Here's how the part is built. I have some questions about the finished solid (model axes, mm). A direction names the side the tool comes from. Give positions to 0.01 mm unless a question says otherwise; leave off trailing zeros. Write each loop counter-clockwise with the first axis right and the second up, starting at its lowest first coordinate (ties: lowest second). Pieces come first, ordered by that corner, then holes. Notation, with made-up numbers: (41, -40) -> (67, -40) arc R17 ccw to (67, -29) -> close; hole circle Ø8 at (70, 25). An arc over 180 degrees is marked (long way). Use CSV: the item, a comma, the result in double quotes. Start each with the question number.
(1) Suppose I cut it at C-C on x = 6.5. List the corners of the cut face in (y, z) for me, plus the area to 3 significant figures.
(2) Suppose I cut it at D-D on z = 2. Give the number of separate pieces and of enclosed holes in the cut face, plus the area to 3 significant figures.
(3) If we mould it in two halves opening along X, with no side actions, what happens to faces 3 (the flat face through (-21.8, -31, 13)), 4 (the flat face through (0, -77.62, 13)), 5 (the flat face through (9, 7.62, 13))? For each: pulls with the +X half, pulls with the -X half, needs draft (parallel to the pull), parting line crosses it, or undercut.
(4) Suppose I cut it at A-A on y = -5.5. List the corners of the cut face in (x, z) for me.
(5) Suppose I cut it at B-B on y = -34. List the corners of the cut face in (x, z) for me, plus the area to 3 significant figures.
(6) Which directions (+Z, -Z, +X, -X, +Y, -Y) give clear straight access to the entire face, cutting with the end or side of a thin tool? Please do faces 1 (the flat face through (9.73, -37.21, 12.52)), 2 (the flat face through (0, 13.97, 13)).
(7) I need wall thicknesses on L1, parallel to X at y = -56.5, z = 21; L2, parallel to Y at x = -13, z = 4; L3, parallel to X at y = 4, z = 7. Which ranges of each line are inside material? Lowest first, please. Write a range as [from, to].
from build123d import *

# Parameters (mm, degrees)
BOSS_EXTRUDE1_DEPTH = 25.4
FILLET1_R           = 0.762


with BuildPart() as part:
    # Sketch1 → Boss-Extrude1 (new body)
    with BuildSketch(Plane.XY):
        Polygon((-21.799999961, -13.97), (-21.799999961, 13.97), (21.799999961, 13.97), (21.799999961, -13.97), (21.799999961, -77.619999954), (-21.799999961, -77.619999954), align=None)
        Polygon((-15.449999961, 7.62), (-2.54, 7.62), (-2.54, 4.572), (-6.6548, 4.572), (-2.933726616, 0.762), (2.933726616, 0.762), (6.6548, 4.572), (2.54, 4.572), (2.54, 7.62), (15.449999961, 7.62), (15.449999961, -7.62), (-15.449999961, -7.62), align=None, mode=Mode.SUBTRACT)
        Polygon((-13.601813914, -20.32), (0, -40.176776526), (13.601813914, -20.32), align=None, mode=Mode.SUBTRACT)
        Polygon((15.449999961, -28.858349607), (3.848460993, -45.794999977), (15.449999961, -62.731650347), align=None, mode=Mode.SUBTRACT)
        Polygon((-3.848460993, -45.794999977), (-15.449999961, -62.731650347), (-15.449999961, -28.858349607), align=None, mode=Mode.SUBTRACT)
        Polygon((0, -51.413223428), (-13.601813914, -71.269999954), (13.601813914, -71.269999954), align=None, mode=Mode.SUBTRACT)
    extrude(amount=BOSS_EXTRUDE1_DEPTH)

    # Fillet1
    fillet1_edges = [part.edges().sort_by_distance(p)[0] for p in [
        (2.54, 7.62, 12.7),
        (2.54, 4.572, 12.7),
        (6.6548, 4.572, 12.7),
        (2.933726616, 0.762, 12.7),
        (-2.933726616, 0.762, 12.7),
        (-6.6548, 4.572, 12.7),
        (-2.54, 4.572, 12.7),
        (-2.54, 7.62, 12.7),
    ]]
    fillet(fillet1_edges, radius=FILLET1_R)


solid = part.part
Geometry says:
1,outline,"(-77.62, 0) -> (-71.27, 0) -> (-71.27, 25.4) -> (-77.62, 25.4) -> close; (-60.9, 0) -> (-49.67, 0) -> (-49.67, 25.4) -> (-60.9, 25.4) -> close; (-41.92, 0) -> (-30.69, 0) -> (-30.69, 25.4) -> (-41.92, 25.4) -> close; (-20.32, 0) -> (-7.62, 0) -> (-7.62, 25.4) -> (-20.32, 25.4) -> close; (7.62, 0) -> (13.97, 0) -> (13.97, 25.4) -> (7.62, 25.4) -> close"
1,area,"1,220 mm²"
2,separate pieces,"1"
2,enclosed holes,"5"
2,area,"2,640 mm²"
3,face 3,"pulls with the -X half"
3,face 4,"needs draft"
3,face 5,"undercut"
4,outline,"(-21.8, 0) -> (-15.45, 0) -> (-15.45, 25.4) -> (-21.8, 25.4) -> close; (15.45, 0) -> (21.8, 0) -> (21.8, 25.4) -> (15.45, 25.4) -> close"
5,outline,"(-21.8, 0) -> (-15.45, 0) -> (-15.45, 25.4) -> (-21.8, 25.4) -> close; (-11.93, 0) -> (-4.23, 0) -> (-4.23, 25.4) -> (-11.93, 25.4) -> close; (4.23, 0) -> (11.93, 0) -> (11.93, 25.4) -> (4.23, 25.4) -> close; (15.45, 0) -> (21.8, 0) -> (21.8, 25.4) -> (15.45, 25.4) -> close"
5,area,"714 mm²"
6,face 1,"+Z, -Z"
6,face 2,"+Z, -Z, +X, -X, +Y"
7,L1,"[-21.8, -15.45], [-11.18, -3.48], [3.48, 11.18], [15.45, 21.8]"
7,L2,"[-77.62, -71.27], [-70.39, -59.15], [-32.44, -21.2], [-20.32, -7.62], [7.62, 13.97]"
7,L3,"[-21.8, -15.45], [-5.58, 5.58], [15.45, 21.8]"
